Can you work these out from the model? Positions are in its coordinate system, mm. Coordinates: 2 decimals unless noted, no trailing zeros. Write each loop counter-clockwise with the first axis right and the second up, starting at its lowest first coordinate (ties: lowest second). Pieces come first, ordered by that corner, then holes. Notation, with made-up numbers: (-35.75, 75.25) - (23.25, 75.25) arc R35 cw to (23.25, 112.25) - close; hole circle Ø3 at (29.25, -11.75). An arc over 180 degrees is marked (long way). Use one line per item in the form item = value. Start each with the question number.
(1) If we section it at A-A on x = 0: Please give me the cut outline in (y, z), then the cut area to 3 significant figures.
(2) If we section it at B-B on x = 25: Please give me the cut outline in (y, z).
(3) If I drill on probe 1 along Y at (x, z) = (25, 1.25); probe 2 along Y at (x, z) = (24, 2.75); probe 3 along Y at (x, z) = (0, 1.25), over which ranges is the centre line in solid material (lowest first)? Write a range as from..to.
(4) If we section it at D-D on z = 0.6: Please give me the cut outline in (x, y), then the cut area to 3 significant figures.
(5) For pin 1 Ø8 at (x, y) = (0.5, 18.5) entering from -Z, with a flat end and sliding along its axis, tell me the tip position at first contact or that it passes through.
(6) If we section it at C-C on y = 7: Please give me the cut outline in (x, z).
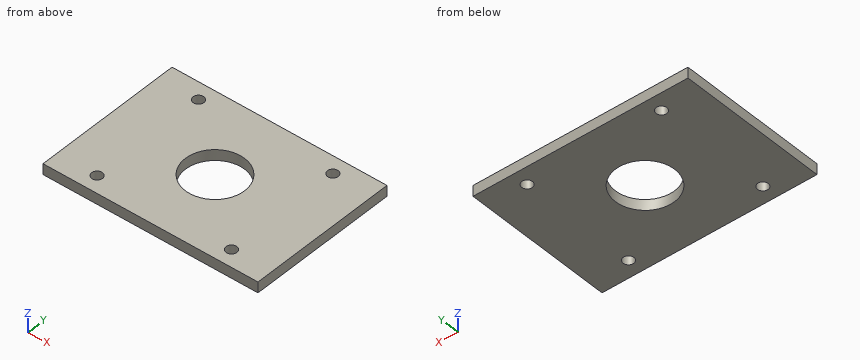
```python
from build123d import *

# Parameters (mm, degrees)
SKETCH_1_W                  = 80
SKETCH_1_H                  = 56
SKETCH_1_R                  = 11
EXTRUDE_1_DEPTH             = 4
SKETCH_2_R                  = 2
CUT_EXTRUDE_1_DEPTH         = 100
PATTERN_LINEAR_1_COUNT      = 2
PATTERN_LINEAR_1_PITCH      = 44
PATTERN_LINEAR_1_COUNT_DIR2 = 2
PATTERN_LINEAR_1_PITCH_DIR2 = 50


with BuildPart() as part:
    # 草图1 → 凸台-拉伸1 (new body)
    with BuildSketch(Plane.XY):
        with Locations((0, 7)):
            Rectangle(SKETCH_1_W, SKETCH_1_H)
        with Locations((0, 7)):
            Circle(SKETCH_1_R, mode=Mode.SUBTRACT)
    extrude(amount=EXTRUDE_1_DEPTH)

    # 草图2 → 切除-拉伸1 (cut)
    with BuildSketch(Plane.XY.offset(4)):
        with Locations((-25, -15)):
            Circle(SKETCH_2_R)
    cut_extrude_1 = extrude(amount=-CUT_EXTRUDE_1_DEPTH, mode=Mode.SUBTRACT)

    # 阵列(线性)1: Cut-Extrude 1 2 × 2
    with Locations(*[(j * PATTERN_LINEAR_1_PITCH_DIR2, i * PATTERN_LINEAR_1_PITCH, 0) for i in range(PATTERN_LINEAR_1_COUNT) for j in range(PATTERN_LINEAR_1_COUNT_DIR2) if (i, j) != (0, 0)]):
        add(cut_extrude_1, mode=Mode.SUBTRACT)


solid = part.part
```
Reported:
q1.outline = (-21, 0) - (-4, 0) - (-4, 4) - (-21, 4) - close; (18, 0) - (35, 0) - (35, 4) - (18, 4) - close
q1.area = 136 mm2
q2.outline = (-21, 0) - (-17, 0) - (-17, 4) - (-21, 4) - close; (-13, 0) - (27, 0) - (27, 4) - (-13, 4) - close; (31, 0) - (35, 0) - (35, 4) - (31, 4) - close
q3.probe_1 = -21..-17, -13..27, 31..35
q3.probe_2 = -21..-16.73, -13.27..27.27, 30.73..35
q3.probe_3 = -21..-4, 18..35
q4.outline = (-40, -21) - (40, -21) - (40, 35) - (-40, 35) - close; hole circle Ø4 at (-25, -15); hole circle Ø4 at (-25, 29); hole circle Ø22 at (0, 7); hole circle Ø4 at (25, -15); hole circle Ø4 at (25, 29)
q4.area = 4,050 mm2
q5.pin_1 = 0
q6.outline = (-40, 0) - (-11, 0) - (-11, 4) - (-40, 4) - close; (11, 0) - (40, 0) - (40, 4) - (11, 4) - close
